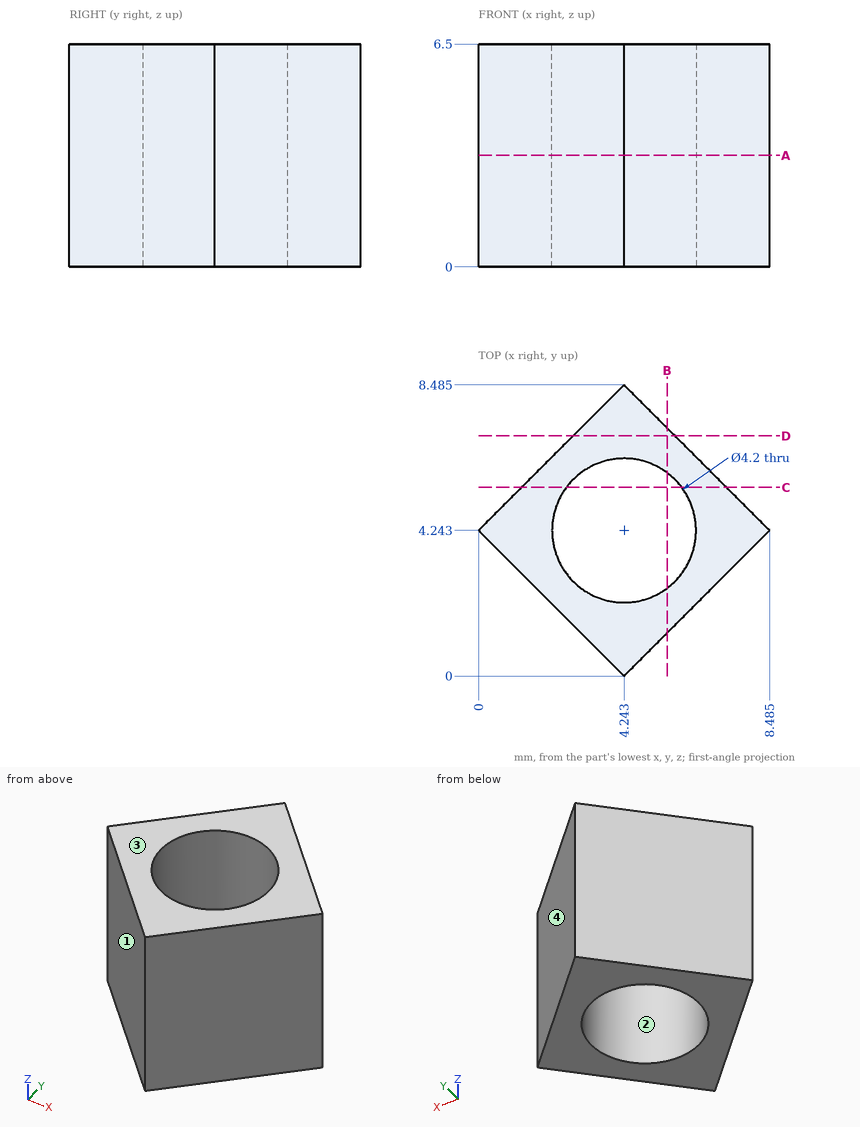
Part print with two shaded views. Sizes in mm from the minimum x, y, z corner. Round coordinates to 2 decimals unless told otherwise and drop trailing zeros. Loops run counter-clockwise (first coordinate to the right, second up) from the corner with the lowest first, then second, coordinate; pieces in that order, holes last.
Item 1: Saw through at D-D (y = 7). List the corners of the cut face in (x, z), then the cut area to 3 significant figures.
Item 2: Two-plate mould, pull along Y, no slides. Class the marked faces 1, 2, 3 and 4: released by +Y, released by -Y, zero draft, split by the parting line, or undercut.
Item 3: Saw through at A-A (z = 3.25). List the corners of the cut face in (x, y) (1 decimal).
Item 4: Pin check, flat tips, straight feed: P1, Ø1, axis at x = 1, z = 2, coming from the +Y side; P2, Ø3, axis at y = 5, z = 4.5, coming from the -X side. Stop position of each tip, or through.
Item 5: Drill centre lines: line 1 along Y through (x, z) = (3.25, 6) (1 decimal); line 2 along Y through (x, z) = (5.5, 2) (1 decimal); line 3 along X through (y, z) = (5, 6.25) (1 decimal). Where is each one in solid material? Low to high.
Item 6: Saw through at B-B (x = 5.5). List the corners of the cut face in (y, z) (1 decimal).
Worked answers:
1. outline: (2.76, 0) - (5.73, 0) - (5.73, 6.5) - (2.76, 6.5) - close
1. area: 19.3 mm2
2. face 1: released by -Y
2. face 2: undercut
2. face 3: zero draft
2. face 4: released by +Y
3. outline: (0, 4.2) - (4.2, 0) - (8.5, 4.2) - (4.2, 8.5) - close; hole circle Ø4.2 at (4.2, 4.2)
4. P1: stops at y = 5.74
4. P2: stops at x = 0
5. line 1: y = 1 to 2.4, 6.1 to 7.5
5. line 2: y = 1.3 to 2.6, 5.9 to 7.2
5. line 3: x = 0.8 to 2.3, 6.2 to 7.7
6. outline: (1.3, 0) - (2.6, 0) - (2.6, 6.5) - (1.3, 6.5) - close; (5.9, 0) - (7.2, 0) - (7.2, 6.5) - (5.9, 6.5) - close
